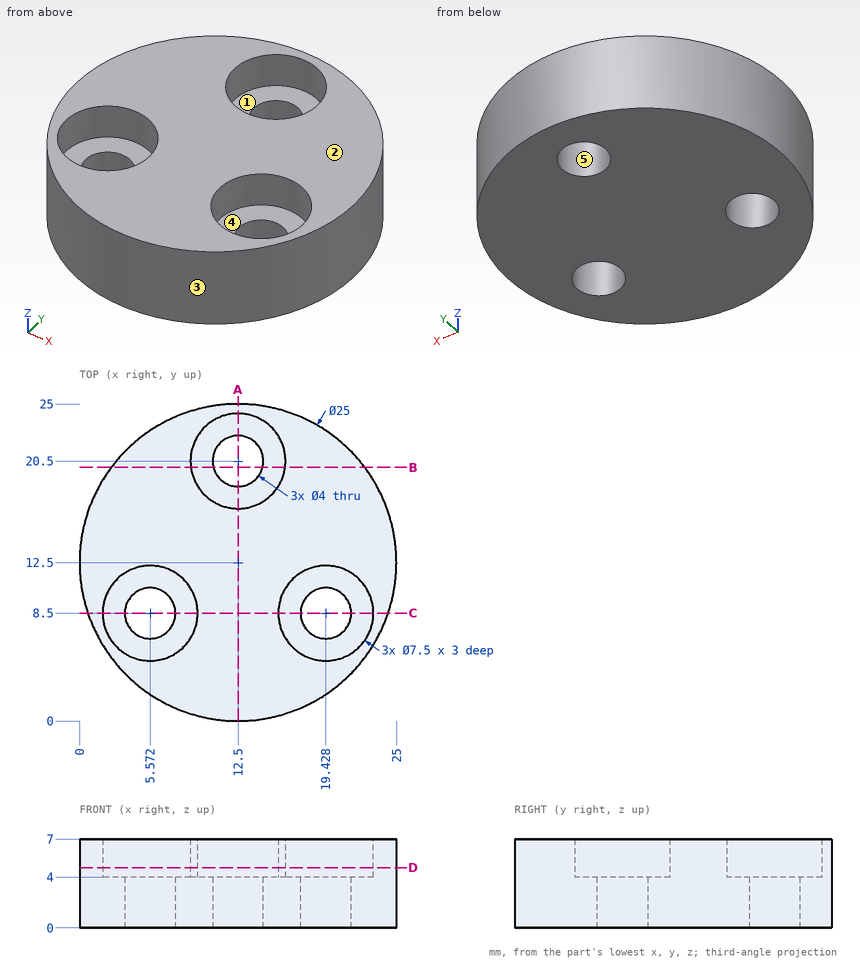
The figure shows three views and two pictorial views of one solid part (mm, origin at its lowest corner). Answer the questions. A direction names the side the tool comes from. Round coordinates to 2 decimals unless told otherwise and drop trailing zeros. Loops run counter-clockwise (first coordinate to the right, second up) from the corner with the lowest first, then second, coordinate; pieces in that order, holes last. Notation, with made-up numbers: (-35.75, 67) - (-7.75, 67) arc R25 cw to (-7.75, 105) - close; hole circle Ø8 at (63.5, -28). An arc over 180 degrees is marked (long way). One line per question, with ' | ' between items. Start each with the question number.
Q1. Section B-B on y = 20 is taken. Give the vertices of the cut face in (x, z), plus the area to 3 significant figures.
Q2. For a pull along Y with two mould halves and no side action, classify the marked faces 1, 2 and 3 as +Y half, -Y half, draft (parallel to the pull), parting line (faces both ways), or undercut.
Q3. Section D-D on z = 4.75 is taken. Give the vertices of the cut face in (x, y), plus the area to 3 significant figures.
Q4. Find the intervals of material crossed by L1, parallel to Y at x = 12.5, z = 2.45; L2, parallel to Y at x = 12.5, z = 4.85; L3, parallel to Z at x = 17, y = 7.25, in increasing order.
Q5. Section C-C on y = 8.5 is taken. Give the vertices of the cut face in (x, z), plus the area to 3 significant figures.
Q6. Section A-A on x = 12.5 is taken. Give the vertices of the cut face in (y, z).
Q7. For the marked faces 4 and 5, determine the directions among +Z, -Z, +X, -X, +Y, -Y from which every point of the face is accessible in a straight line to the end or side of a thin tool.
Q8. Flat-ended cylindrical pins translate along their axes: pin 1 (4 mm diameter, centred on x = 8, z = 0.5, fed in from -Y); pin 2 (2 mm diameter, centred on x = 18.5, y = 7.5, fed in from +Z); pin 3 (1 mm diameter, centred on y = 15, z = 3, fed in from -X). Find the tip coordinate at first contact, or state that the pin passes through.
Established:
1) outline: (2.5, 0) - (10.56, 0) - (10.56, 4) - (8.78, 4) - (8.78, 7) - (2.5, 7) - close; (14.44, 0) - (22.5, 0) - (22.5, 7) - (16.22, 7) - (16.22, 4) - (14.44, 4) - close | area: 102 mm²
2) face 1: undercut | face 2: draft | face 3: parting line
3) outline: circle Ø25 at (12.5, 12.5); hole circle Ø7.5 at (5.57, 8.5); hole circle Ø7.5 at (12.5, 20.5); hole circle Ø7.5 at (19.43, 8.5) | area: 358 mm²
4) L1: 0 to 18.5, 22.5 to 25 | L2: 0 to 16.75, 24.25 to 25 | L3: 0 to 4
5) outline: (0.66, 0) - (3.57, 0) - (3.57, 4) - (1.82, 4) - (1.82, 7) - (0.66, 7) - close; (7.57, 0) - (17.43, 0) - (17.43, 4) - (15.68, 4) - (15.68, 7) - (9.32, 7) - (9.32, 4) - (7.57, 4) - close; (21.43, 0) - (24.34, 0) - (24.34, 7) - (23.18, 7) - (23.18, 4) - (21.43, 4) - close | area: 88.8 mm²
6) outline: (0, 0) - (18.5, 0) - (18.5, 4) - (16.75, 4) - (16.75, 7) - (0, 7) - close; (22.5, 0) - (25, 0) - (25, 7) - (24.25, 7) - (24.25, 4) - (22.5, 4) - close
7) face 4: +Z | face 5: +Z, -Z
8) pin 1: y = 0.25 | pin 2: z = 4 | pin 3: x = 0.16
